For this review, take the finished solid that the model builds, in its own axes (mm). Face numbers are marked on the shaded views. Round coordinates to 2 decimals unless told otherwise and drop trailing zeros. Write each loop counter-clockwise with the first axis right and the second up, starting at its lowest first coordinate (ties: lowest second). Pieces come first, ordered by that corner, then holes. Notation, with made-up numbers: (-21.5, 65) -> (-9.5, 65) arc R17 cw to (-9.5, 98) -> close; hole circle Ø10 at (37, -12). An arc over 180 degrees is marked (long way). Answer in a Markdown table with one row per item. Add a question column.
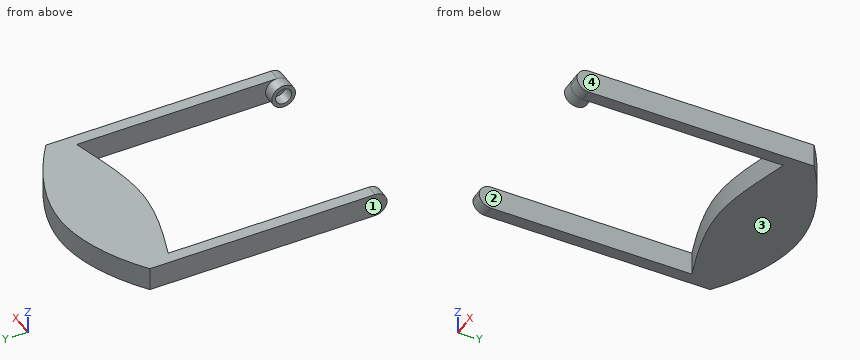
```python
from build123d import *

# Parameters (mm, degrees)
EXTRUDE_1_DEPTH          = 6
CUT_EXTRUDE_1_DEPTH      = 86.959139
CUT_EXTRUDE_1_DEPTH_BACK = 86.959139
SKETCH_3_R               = 2.05
EXTRUDE_2_DEPTH          = 3


with BuildPart() as part:
    # 草图1 → 凸台-拉伸1 (new body)
    with BuildSketch(Plane.XY):
        with BuildLine():
            Line((0, 0), (0, 60))
            add(Edge.make_bspline(
                [(0, 60), (6.932027, 65.303268), (25.02154, 74.137336), (42.974448, 65.073065), (50, 60)],
                knots=[0, 0, 0, 0, 0.50035, 1, 1, 1, 1], degree=3))
            Line((50, 60), (50, 0))
            Line((50, 0), (47, 0))
            Line((47, 0), (47, 53.774366))
            add(Edge.make_bspline(
                [(3, 53.774366), (9.965867, 51.405734), (25.033485, 46.45053), (39.925766, 51.813875), (47, 53.774366)],
                knots=[0, 0, 0, 0, 0.500345, 1, 1, 1, 1], degree=3))
            Line((3, 53.774366), (3, 0))
            Line((3, 0), (0, 0))
        make_face()
    extrude(amount=EXTRUDE_1_DEPTH)

    # 草图2 → 切除-拉伸1 (cut, two sides: drawn at the far end of the back side and taken through both)
    with BuildSketch(Plane.ZY.offset(-CUT_EXTRUDE_1_DEPTH_BACK)):
        with BuildLine():
            Line((0, 0), (3, 0))
            ThreePointArc((3, 0), (0.87868, 0.87868), (0, 3))
            Line((0, 3), (0, 0))
        make_face()
        with BuildLine():
            Line((6, 0), (6, 3))
            ThreePointArc((6, 3), (5.12132, 0.87868), (3, 0))
            Line((3, 0), (6, 0))
        make_face()
    extrude(amount=CUT_EXTRUDE_1_DEPTH + CUT_EXTRUDE_1_DEPTH_BACK, mode=Mode.SUBTRACT)

    # 草图3 → 凸台-拉伸2 (add)
    with BuildSketch(Plane.ZY.offset(-47)):
        with BuildLine():
            ThreePointArc((6, 3), (3, 6), (0, 3))
            ThreePointArc((0, 3), (3, 0), (6, 3))
        make_face()
        with Locations(Location((3, 3, 0), (0, 0, 270))):
            Circle(SKETCH_3_R, mode=Mode.SUBTRACT)
    extrude(amount=EXTRUDE_2_DEPTH)


solid = part.part
```
1. Clearance check with flat-ended pins moving along their axes: pin 1 Ø1.8 at (y, z) = (25, 2) entering from -X; pin 2 Ø8 at (x, y) = (8, 41.5) entering from +Z; pin 3 Ø2 at (x, z) = (44.5, 0.5) entering from -Y; pin 4 Ø1.5 at (x, z) = (8.5, 2.5) entering from +Y. State where each tip first meets the part, or that it passes through.
2. The part is to be moulded in two halves that separate along X. For the marked faces 1, 2, 3 and 4, say which applies: pulls with the +X half, pulls with the -X half, needs draft (parallel to the pull), parting line crosses it, or undercut.
3. We need section A-A (y = 29.5). Write out the cut boundary in (x, z), plus the area to 3 significant figures.
4. For L1, parallel to X at y = 20.5, z = 4; L2, parallel to Z at x = 44.75, y = 3; L3, parallel to Y at x = 24.5, z = 2.5, list the stretches that pass through material, from the lowest coordinate up. Write a range as [from, to].
Response:
| question | item | result |
|---|---|---|
| 1 | pin 1 | x = 0 |
| 1 | pin 2 | through |
| 1 | pin 3 | y = 0.4 |
| 1 | pin 4 | y = 65.74 |
| 2 | face 1 | pulls with the -X half |
| 2 | face 2 | undercut |
| 2 | face 3 | needs draft |
| 2 | face 4 | pulls with the +X half |
| 3 | outline | (0, 0) -> (3, 0) -> (3, 6) -> (0, 6) -> close; (47, 0) -> (50, 0) -> (50, 6) -> (47, 6) -> close |
| 3 | area | 36.0 mm2 |
| 4 | L1 | [0, 3], [47, 50] |
| 4 | L2 | [0, 0.95], [5.05, 6] |
| 4 | L3 | [49.03, 69.66] |
